For this review, take the finished solid that the model builds, in its own axes (mm). A direction names the side the tool comes from. Coordinates: 2 decimals unless noted, no trailing zeros. Write each loop counter-clockwise with the first axis right and the second up, starting at its lowest first coordinate (ties: lowest second). Pieces come first, ordered by that corner, then holes. Notation, with made-up numbers: (-28.5, 21) - (-7.5, 21) arc R10 ccw to (-7.5, 26) - close; hole circle Ø3 at (78, 65). An arc over 180 degrees is marked (long way). Write each question's results on one line, items separated by ' | '.
from build123d import *

# Parameters (mm, degrees)
SKETCH2_W           = 20
SKETCH2_H           = 13
BOSS_EXTRUDE1_DEPTH = 2
BOSS_EXTRUDE2_DEPTH = 2
SKETCH4_W           = 11
SKETCH4_H           = 8
BOSS_EXTRUDE3_DEPTH = 1
SKETCH5_R           = 2
CUT_EXTRUDE1_DEPTH  = 6


with BuildPart() as part:
    # Sketch2 → Boss-Extrude1 (new body)
    with BuildSketch(Plane(origin=(0, 0, 0), x_dir=(1, 0, 0), z_dir=(0, 1, 0))):
        with Locations((10, 6.5)):
            Rectangle(SKETCH2_W, SKETCH2_H)
    extrude(amount=BOSS_EXTRUDE1_DEPTH)

    # Sketch3 → Boss-Extrude2 (add)
    with BuildSketch(Plane.XY):
        Polygon((0, 0), (20, 0), (20, 10), (9.534028741, 10), (0, 2), align=None)
    boss_extrude2 = extrude(amount=BOSS_EXTRUDE2_DEPTH)

    # Mirror1: Boss-Extrude2 across plane
    add(boss_extrude2.mirror(Plane.XY.offset(-5.5)))

    # Sketch4 → Boss-Extrude3 (add)
    with BuildSketch(Plane(origin=(20, 0, 0), x_dir=(0, 0, -1), z_dir=(1, 0, 0))):
        with Locations((5.5, 6)):
            Rectangle(SKETCH4_W, SKETCH4_H)
    extrude(amount=-BOSS_EXTRUDE3_DEPTH)

    # Sketch5 → Cut-Extrude1 (cut)
    with BuildSketch(Plane(origin=(20, 0, 0), x_dir=(0, 0, -1), z_dir=(1, 0, 0))):
        with Locations((5.5, 5)):
            Circle(SKETCH5_R)
    extrude(amount=-CUT_EXTRUDE1_DEPTH, mode=Mode.SUBTRACT)


solid = part.part
Q1. Wall thickness on line 1 along Z through (x, y) = (8.75, 4.25); line 2 along Y through (x, z) = (19.4, -5.5); line 3 along Y through (x, z) = (2.75, -7.75): over which ranges is each line inside the solid? List them lowest first. Write a range as from..to.
Results found:
line 1: -13..-11, 0..2 | line 2: 0..3, 7..10 | line 3: 0..2
Q2. Take a section at A-A on z = -5.5. State the section outline as (x, y) points.
Results found:
outline: (0, 0) - (20, 0) - (20, 3) - (19, 3) - (19, 2) - (0, 2) - close; (19, 7) - (20, 7) - (20, 10) - (19, 10) - close
Q3. Take a section at B-B on y = 5. State the section outline as (x, z) points.
Results found:
outline: (3.58, -13) - (20, -13) - (20, -7.5) - (19, -7.5) - (19, -11) - (3.58, -11) - close; (3.58, 0) - (19, 0) - (19, -3.5) - (20, -3.5) - (20, 2) - (3.58, 2) - close
Q4. Take a section at C-C on x = 15.75. State the section outline as (y, z) points, plus the area to 3 significant figures.
Results found:
outline: (0, -13) - (10, -13) - (10, -11) - (2, -11) - (2, 0) - (10, 0) - (10, 2) - (0, 2) - close | area: 62.0 mm2
Q5. Take a section at D-D on z = -8. State the section outline as (x, y) points.
Results found:
outline: (0, 0) - (20, 0) - (20, 10) - (19, 10) - (19, 2) - (0, 2) - close
Q6. For faces 1 (the face through (12, 5, -13)), 2 (the face through (19, 7, -4)), list the 3-axis set-ups (+Z, -Z, +X, -X, +Y, -Y) from which the entire face can be reached by the end or side of a thin tool; tool diameter is ignored.
Results found:
face 1: -Z, +X, -X, +Y, -Y | face 2: -X, +Y
Q7. For pin 1 (3 mm diameter, centred on x = 3.5, z = -8, fed in from +Y); pin 2 (4 mm diameter, centred on y = 8, z = -8.5, fed in from -X), all flat-tipped, find the tip position at first contact; note any pin that passes through.
Results found:
pin 1: y = 2 | pin 2: x = 19
Q8. Mouldability with a two-part tool opening along X and no side actions: class faces 3 (the face through (20, 6.2, -3.7)), 4 (the face through (19.8, 10, -5.5)), 5 (the face through (4.834, 6.056, -11.986)) as pulls with the +X half, pulls with the -X half, needs draft (parallel to the pull), parting line crosses it, or undercut.
Results found:
face 3: pulls with the +X half | face 4: needs draft | face 5: pulls with the -X half
